```python
from build123d import *

# Parameters (mm, degrees)
BOSS_EXTRUDE1_DEPTH = 5.08
FILLET1_R           = 1.27


with BuildPart() as part:
    # Sketch1 → Boss-Extrude1 (new body)
    with BuildSketch(Plane(origin=(0, 0, 0), x_dir=(1, 0, 0), z_dir=(0, 1, 0))):
        Polygon((5.08, 0), (10.16, 0), (10.16, 5.08), (-5.08, 5.08), (-5.08, 0), (0, 0), (0, -2.54), (5.08, -2.54), align=None)
    extrude(amount=BOSS_EXTRUDE1_DEPTH)

    # Fillet1
    fillet1_edges = [part.edges().sort_by_distance(p)[0] for p in [
        (-5.08, 2.54, 0),
        (-5.08, 2.54, -5.08),
        (10.16, 2.54, -5.08),
        (10.16, 2.54, 0),
    ]]
    fillet(fillet1_edges, radius=FILLET1_R)


solid = part.part
```
Part model, mm, in its own coordinate system. A direction names the side the tool comes from. Coordinates: 2 decimals unless noted, no trailing zeros. Loops run counter-clockwise (first coordinate to the right, second up) from the corner with the lowest first, then second, coordinate; pieces in that order, holes last. Notation, with made-up numbers: (-24.5, 48.25) - (30.5, 48.25) arc R28 ccw to (30.5, 78.25) - close; hole circle Ø7 at (48.5, 88). An arc over 180 degrees is marked (long way). Write item = value, one per line. Start each with the question number.
Item 1: Flat gauge pins, fed straight in: pin 1 Ø3 at (x, y) = (7, 2) entering from +Z; pin 2 Ø0.8 at (y, z) = (2, 1.5) entering from -X; pin 3 Ø0.8 at (y, z) = (4, 0.5) entering from +X. Where does each tip first touch, or does it go through?
Item 2: Cut at A-A, the plane y = 3.4. Give the cut face in (x, z).
Item 3: Cut at B-B, the plane x = -1.5. Give the cut face in (y, z).
Item 4: Cut at C-C, the plane z = 0.5. Give the cut face in (x, y), and give its area (3 significant figures).
Item 5: 3-axis set-ups, long thin cutter, end or side, ignore diameter. For faces 4 (the flat face through (-2, 3, 0)), 5 (the flat face through (3, 3, -5.08)), 6 (the flat face through (7, 3, 0)): which of +Z, -Z, +X, -X, +Y, -Y reach the whole face in a straight line?
Item 6: Wall check: L1, parallel to Z at x = -1.75, y = 1.1; L2, parallel to X at y = 4.75, z = 1; L3, parallel to X at y = 3.6, z = -4. Give the ranges that are in metal, low to high. Write a range as from..to.
Item 7: Mould opens along X. For faces 1 (the cylindrical face through (9.778, 2.576, -0.362)), 2 (the flat face through (2, 5.08, -2)), 3 (the flat face through (0, 3, 1)) say: released by +X, released by -X, zero draft, split by the parting line, or undercut.
The answers:
q1.pin_1 = 0
q1.pin_2 = 0
q1.pin_3 = 5.08
q2.outline = (-5.08, -3.81) arc R1.27 ccw to (-3.81, -5.08) - (8.89, -5.08) arc R1.27 ccw to (10.16, -3.81) - (10.16, -1.27) arc R1.27 ccw to (8.89, 0) - (5.08, 0) - (5.08, 2.54) - (0, 2.54) - (0, 0) - (-3.81, 0) arc R1.27 ccw to (-5.08, -1.27) - close
q3.outline = (0, -5.08) - (5.08, -5.08) - (5.08, 0) - (0, 0) - close
q4.outline = (0, 0) - (5.08, 0) - (5.08, 5.08) - (0, 5.08) - close
q4.area = 25.8 mm2
q5.face_4 = +Z, -X, +Y, -Y
q5.face_5 = -Z, +X, -X, +Y, -Y
q5.face_6 = +Z, +X, +Y, -Y
q6.L1 = -5.08..0
q6.L2 = 0..5.08
q6.L3 = -5.07..10.15
q7.face_1 = released by +X
q7.face_2 = zero draft
q7.face_3 = released by -X
